Autodesk Fusion 360 part; units mm, degrees
sketch "Sketch1" plane through (0, 0, 0) normal (0, 0, 1) x (1, 0, 0)
  line L0 (-20, 95) -> (20, 95)
  line L1 (20, 95) -> (20, 0)
  line L2 (20, 0) -> (-20, 0)
  line L3 (-20, 0) -> (-20, 95)
  circle A0 centre (-10, 80) radius 2
  circle A1 centre (10, 80) radius 2
  circle A2 centre (-10, 50) radius 2
  circle A3 centre (10, 50) radius 2
  line L4 (0, 125) -> (0, -25) construction
  dimension "d1" = 95
  dimension "d2" = 40
  dimension "d3" = 4
  dimension "d8" = 20
  dimension "d9" = -30
  dimension "d10" = 15
extrude "Extrude1" add sketch "Sketch1" along normal blind 2 makes body 1
ref_plane "WorkPlane1" through (0, 0, 0) normal (0, 0.7071, -0.7071) x (-1, 0, 0)
mirror "Mirror1" about plane through (0, 0, 0) normal (0, 0.7071, -0.7071) of "Extrude1" makes body 2
combine "Combine1" operation add target body 2 tool bodies 1
For this review, take the finished solid that the model builds, in its own axes (mm). A direction names the side the tool comes from. Round coordinates to 2 decimals unless told otherwise and drop trailing zeros. Order: outer loops, then holes, each group sorted by start corner. A loop starts at its lowest first (then second) coordinate and runs counter-clockwise, first axis right, second up. Notation, with made-up numbers: (-15.5, 38) -> (-3.5, 38) arc R31 ccw to (-3.5, 74) -> close; hole circle Ø1 at (-13, 76). An arc over 180 degrees is marked (long way). Write item = value, one per line. Start each with the question number.
1) Take a section at A-A on x = 10. State the section outline as (y, z) points, plus the area to 3 significant figures.
2) Take a section at B-B on z = 50. State the section outline as (x, y) points.
3) To check wall thickness, follow line 1 (Y direction, x = 10, z = 1.4); line 2 (Y direction, x = 0.5, z = 15). State the ranges of each line that lie inside material, in increasing order. Write a range as from..to.
4) Insertion check: pin 1 (2.5 mm diameter, centred on x = -10, y = 50, fed in from -Z); pin 2 (8 mm diameter, centred on x = 2, y = 79, fed in from +Z); pin 3 (5 mm diameter, centred on x = -10, z = 50, fed in from +Y). Each pin has a flat end and moves straight along its axis. Give the tip position at first contact, or say it passes through.
5) The part is to be moulded in two halves that separate along X. For faces 3 (the face through (-10, 1, 82)), 4 (the face through (0, 0, 48)), 5 (the face through (20, 1.5, 26.2)), say which applies: +X half, -X half, draft (parallel to the pull), parting line (faces both ways), or undercut.
6) Take a section at D-D on x = 1.5. State the section outline as (y, z) points.
7) Tool access review of faces 1 (the face through (0, 47, 0)), 2 (the face through (0, 49, 2)): name each direction out of +Z, -Z, +X, -X, +Y, -Y from which nothing blocks a thin tool from reaching the whole face with its end or side.
Verdict:
q1.outline = (0, 0) -> (48, 0) -> (48, 2) -> (2, 2) -> (2, 48) -> (0, 48) -> close; (0, 52) -> (2, 52) -> (2, 78) -> (0, 78) -> close; (0, 82) -> (2, 82) -> (2, 95) -> (0, 95) -> close; (52, 0) -> (78, 0) -> (78, 2) -> (52, 2) -> close; (82, 0) -> (95, 0) -> (95, 2) -> (82, 2) -> close
q1.area = 344 mm2
q2.outline = (-20, 0) -> (-12, 0) -> (-12, 2) -> (-20, 2) -> close; (-8, 0) -> (8, 0) -> (8, 2) -> (-8, 2) -> close; (12, 0) -> (20, 0) -> (20, 2) -> (12, 2) -> close
q3.line_1 = 0..48, 52..78, 82..95
q3.line_2 = 0..2
q4.pin_1 = through
q4.pin_2 = 2
q4.pin_3 = 2
q5.face_3 = undercut
q5.face_4 = draft
q5.face_5 = +X half
q6.outline = (0, 0) -> (95, 0) -> (95, 2) -> (2, 2) -> (2, 95) -> (0, 95) -> close
q7.face_1 = -Z, +X, -X, +Y, -Y
q7.face_2 = +Z, +X, -X, +Y
